The model under review builds one solid part; all positions refer to its coordinate system, in mm. Round coordinates to 2 decimals unless told otherwise and drop trailing zeros. Write each loop counter-clockwise with the first axis right and the second up, starting at its lowest first coordinate (ties: lowest second). Pieces come first, ordered by that corner, then holes. Notation, with made-up numbers: (45.25, -39.5) - (70.25, -39.5) arc R18 ccw to (70.25, -17.5) - close; hole circle Ø2 at (16, 25.25). An arc over 180 degrees is marked (long way). Return JSON: item names as keys, results as strings.
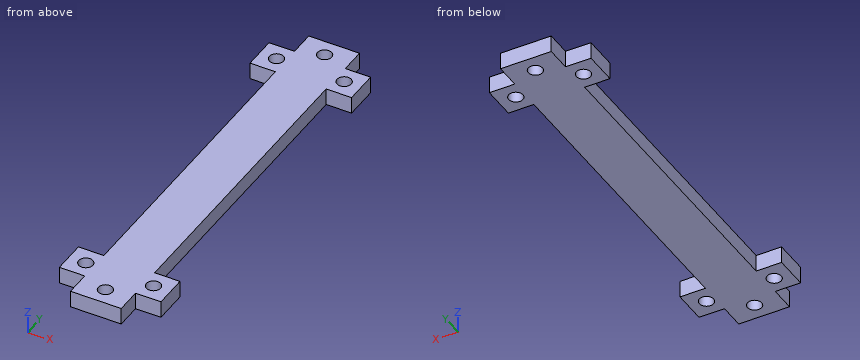
from build123d import *

# Parameters (mm, degrees)
SKETCH1_W           = 15
SKETCH1_H           = 90
SKETCH1_R           = 2.1
SKETCH1_H_2         = 7.5
BOSS_EXTRUDE1_DEPTH = 5


with BuildPart() as part:
    # Sketch1 → Boss-Extrude1 (new body)
    with BuildSketch(Plane.XY):
        with Locations((7.5, 45)):
            Rectangle(SKETCH1_W, SKETCH1_H)
        Polygon((-7.5, 90), (0, 90), (15, 90), (22.5, 90), (22.5, 100), (15, 100), (0, 100), (-7.5, 100), align=None)
        with Locations((-2.5, 95)):
            Circle(SKETCH1_R, mode=Mode.SUBTRACT)
        with Locations((17.5, 95)):
            Circle(SKETCH1_R, mode=Mode.SUBTRACT)
        with Locations((7.5, 103.75)):
            Rectangle(SKETCH1_W, SKETCH1_H_2)
        with Locations((7.5, 102.5)):
            Circle(SKETCH1_R, mode=Mode.SUBTRACT)
        Polygon((15, 0), (0, 0), (-7.5, 0), (-7.5, -10), (0, -10), (15, -10), (22.5, -10), (22.5, 0), align=None)
        with Locations((-2.5, -5)):
            Circle(SKETCH1_R, mode=Mode.SUBTRACT)
        with Locations((17.5, -5)):
            Circle(SKETCH1_R, mode=Mode.SUBTRACT)
        with Locations((7.5, -13.75)):
            Rectangle(SKETCH1_W, SKETCH1_H_2)
        with Locations((7.5, -12.5)):
            Circle(SKETCH1_R, mode=Mode.SUBTRACT)
    extrude(amount=BOSS_EXTRUDE1_DEPTH)


solid = part.part
(1) Add section D-D (x = 17.5). Write out the cut boundary in (y, z).
Filled in:
{"outline": "(-10, 0) - (-7.1, 0) - (-7.1, 5) - (-10, 5) - close; (-2.9, 0) - (0, 0) - (0, 5) - (-2.9, 5) - close; (90, 0) - (92.9, 0) - (92.9, 5) - (90, 5) - close; (97.1, 0) - (100, 0) - (100, 5) - (97.1, 5) - close"}
(2) Clearance check with flat-ended pins moving along their axes: pin 1 Ø2.5 at (x, z) = (-5, 3.5) entering from -Y; pin 2 Ø2.5 at (y, z) = (64.5, 3) entering from -X. State where each tip first meets the part, or that it passes through.
Filled in:
{"pin 1": "stops at y = -10", "pin 2": "stops at x = 0"}
(3) Wall thickness on line 1 (Y direction, x = -2.5, z = 2); line 2 (Y direction, x = 7.5, z = 3.2); line 3 (X direction, y = -3.5, z = 3.7): over which ranges is each line inside the solid? List them lowest first.
Filled in:
{"line 1": "y = -10 to -7.1, -2.9 to 0, 90 to 92.9, 97.1 to 100", "line 2": "y = -17.5 to -14.6, -10.4 to 100.4, 104.6 to 107.5", "line 3": "x = -7.5 to -3.97, -1.03 to 16.03, 18.97 to 22.5"}
(4) Add section C-C (z = 2.8). Write out the cut boundary in (x, y), plus the area to 3 significant figures.
Filled in:
{"outline": "(-7.5, -10) - (0, -10) - (0, -17.5) - (15, -17.5) - (15, -10) - (22.5, -10) - (22.5, 0) - (15, 0) - (15, 90) - (22.5, 90) - (22.5, 100) - (15, 100) - (15, 107.5) - (0, 107.5) - (0, 100) - (-7.5, 100) - (-7.5, 90) - (0, 90) - (0, 0) - (-7.5, 0) - close; hole circle Ø4.2 at (-2.5, -5); hole circle Ø4.2 at (-2.5, 95); hole circle Ø4.2 at (7.5, -12.5); hole circle Ø4.2 at (7.5, 102.5); hole circle Ø4.2 at (17.5, -5); hole circle Ø4.2 at (17.5, 95)", "area": "2,090 mm2"}
(5) Add section A-A (x = 7.5). Write out the cut boundary in (y, z), plus the area to 3 significant figures.
Filled in:
{"outline": "(-17.5, 0) - (-14.6, 0) - (-14.6, 5) - (-17.5, 5) - close; (-10.4, 0) - (100.4, 0) - (100.4, 5) - (-10.4, 5) - close; (104.6, 0) - (107.5, 0) - (107.5, 5) - (104.6, 5) - close", "area": "583 mm2"}
(6) Add section B-B (y = 102.5). Write out the cut boundary in (x, z), plus the area to 3 significant figures.
Filled in:
{"outline": "(0, 0) - (5.4, 0) - (5.4, 5) - (0, 5) - close; (9.6, 0) - (15, 0) - (15, 5) - (9.6, 5) - close", "area": "54.0 mm2"}
